Geometry: final body of the model. Coordinates: model frame, mm. Face numbers are marked on the shaded views. A direction names the side the tool comes from. Round coordinates to 2 decimals unless told otherwise and drop trailing zeros. Order: outer loops, then holes, each group sorted by start corner. A loop starts at its lowest first (then second) coordinate and runs counter-clockwise, first axis right, second up. Notation, with made-up numbers: (-5, 87) - (17, 87) arc R21 ccw to (17, 122) - close; hole circle Ø7 at (66, -33). An arc over 180 degrees is marked (long way). Put each result on its own line as item: value. Start each with the question number.
(1) Material intervals for L1, parallel to X at y = 3.35, z = 38.5; L2, parallel to Y at x = -114, z = 46.5; L3, parallel to X at y = 4, z = 41.25, sorted ascending. Write a range as [from, to].
(2) Section B-B (z = 43). Output: boundary loops of the cut face in (x, y).
(3) Pull-direction query (X, two-part tool) for the marked faces 3, 4 and 5; classes: released by +X, released by -X, zero draft, split by the parting line, or undercut.
(4) Section A-A (y = 3.95). Count the separate pieces of the cut face and the enclosed holes in it, and give its area (3 significant figures).
(5) Access query for the marked faces 1 and 2. Directions: +Z, -Z, +X, -X, +Y, -Y. A direction counts if a zero-diameter tool reaches every point of the face in a straight line with its end or side. Return the directions, or none.
(6) Pin query (flat end, axial travel): P1, Ø10, axis at x = -105, z = 35.5, coming from the +Y side. Return the tip coordinate at first contact, or that it passes through.
(7) Section C-C (x = -100). Output: boundary loops of the cut face in (y, z), and give its area (3 significant figures).
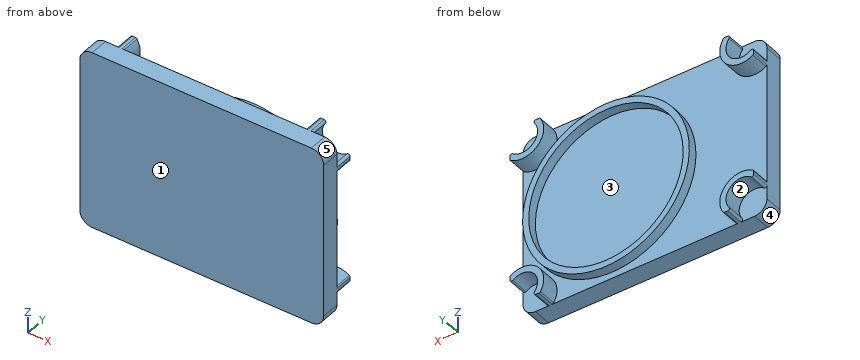
from build123d import *

# Parameters (mm, degrees)
SKETCH1_W           = 39.5
SKETCH1_H           = 29
BOSS_EXTRUDE1_DEPTH = 3
SKETCH2_R           = 13.5
SKETCH2_R_2         = 12.5
BOSS_EXTRUDE3_DEPTH = 1.5
BOSS_EXTRUDE4_DEPTH = 3
FILLET1_R           = 2
FILLET2_R           = 0.3


with BuildPart() as part:
    # Sketch1 → Boss-Extrude1 (new body)
    with BuildSketch(Plane(origin=(0, 0, 0), x_dir=(1, 0, 0), z_dir=(0, 1, 0))):
        with Locations((-109.95705295, -40.158748639)):
            Rectangle(SKETCH1_W, SKETCH1_H)
    extrude(amount=BOSS_EXTRUDE1_DEPTH)

    # Sketch2 → Boss-Extrude3 (add)
    with BuildSketch(Plane(origin=(0, 3, 0), x_dir=(1, 0, 0), z_dir=(0, 1, 0))):
        with Locations(Location((-104.70705295, -40.158748639, 0), (0, 0, 270))):
            Circle(SKETCH2_R)
        with Locations(Location((-104.70705295, -40.158748639, 0), (0, 0, 270))):
            Circle(SKETCH2_R_2, mode=Mode.SUBTRACT)
    extrude(amount=BOSS_EXTRUDE3_DEPTH)

    # Sketch3 → Boss-Extrude4 (add)
    with BuildSketch(Plane(origin=(0, 3, 0), x_dir=(1, 0, 0), z_dir=(0, 1, 0))):
        with BuildLine():
            Line((-124.834771627, -25.658748639), (-126.20705295, -25.658748639))
            ThreePointArc((-126.20705295, -25.658748639), (-125.939285997, -29.426515592), (-129.70705295, -29.158748639))
            Line((-129.70705295, -29.158748639), (-129.70705295, -30.531029962))
            ThreePointArc((-129.70705295, -30.531029962), (-125.232179216, -30.133622373), (-124.834771627, -25.658748639))
        make_face()
        with BuildLine():
            Line((-93.70705295, -25.658748639), (-95.079334273, -25.658748639))
            ThreePointArc((-95.079334273, -25.658748639), (-94.681926684, -30.133622373), (-90.20705295, -30.531029962))
            Line((-90.20705295, -30.531029962), (-90.20705295, -29.158748639))
            ThreePointArc((-90.20705295, -29.158748639), (-93.974819903, -29.426515592), (-93.70705295, -25.658748639))
        make_face()
        with BuildLine():
            ThreePointArc((-124.834771627, -54.658748639), (-125.232179216, -50.183874905), (-129.70705295, -49.786467316))
            Line((-129.70705295, -49.786467316), (-129.70705295, -51.158748639))
            ThreePointArc((-129.70705295, -51.158748639), (-125.939285997, -50.890981686), (-126.20705295, -54.658748639))
            Line((-126.20705295, -54.658748639), (-124.834771627, -54.658748639))
        make_face()
        with BuildLine():
            Line((-90.20705295, -51.158748639), (-90.20705295, -49.786467316))
            ThreePointArc((-90.20705295, -49.786467316), (-94.681926684, -50.183874905), (-95.079334273, -54.658748639))
            Line((-95.079334273, -54.658748639), (-93.70705295, -54.658748639))
            ThreePointArc((-93.70705295, -54.658748639), (-93.974819903, -50.890981686), (-90.20705295, -51.158748639))
        make_face()
    extrude(amount=BOSS_EXTRUDE4_DEPTH)

    # Fillet1
    fillet1_edges = [part.edges().sort_by_distance(p)[0] for p in [
        (-129.70705295, 1.5, 25.658748639),
        (-90.20705295, 1.5, 25.658748639),
        (-90.20705295, 1.5, 54.658748639),
        (-129.70705295, 1.5, 54.658748639),
    ]]
    fillet(fillet1_edges, radius=FILLET1_R)

    # Fillet2
    fillet2_edges = [part.edges().sort_by_distance(p)[0] for p in [
        (-93.70705295, 4.5, 54.658748639),
        (-90.20705295, 4.5, 51.158748639),
        (-90.20705295, 4.5, 49.786467316),
        (-95.079334273, 4.5, 54.658748639),
        (-126.20705295, 4.5, 54.658748639),
        (-124.834771627, 4.5, 54.658748639),
        (-129.70705295, 4.5, 49.786467316),
        (-129.70705295, 4.5, 51.158748639),
        (-93.70705295, 4.5, 25.658748639),
        (-95.079334273, 4.5, 25.658748639),
        (-90.20705295, 4.5, 30.531029962),
        (-90.20705295, 4.5, 29.158748639),
        (-129.70705295, 4.5, 29.158748639),
        (-129.70705295, 4.5, 30.531029962),
        (-124.834771627, 4.5, 25.658748639),
        (-126.20705295, 4.5, 25.658748639),
    ]]
    fillet(fillet2_edges, radius=FILLET2_R)


solid = part.part
Checks:
1. L1: x = [-118.1, -117.1], [-92.32, -91.31]
1. L2: y = [0, 3]
1. L3: x = [-118.16, -117.16], [-92.25, -91.25]
2. outline: (-129.71, 0) - (-90.21, 0) - (-90.21, 3) - (-91.51, 3) - (-91.51, 4.5) - (-92.53, 4.5) - (-92.53, 3) - (-116.88, 3) - (-116.88, 4.5) - (-117.9, 4.5) - (-117.9, 3) - (-129.71, 3) - close
3. face 3: undercut
3. face 4: released by -X
3. face 5: released by +X
4. separate pieces: 5
4. enclosed holes: 1
4. area: 117 mm²
5. face 1: +Z, -Z, +X, -X, -Y
5. face 2: +Y
6. P1: stops at y = 3
7. outline: (0, 25.66) - (3, 25.66) - (3, 27.51) - (4.5, 27.51) - (4.5, 28.58) - (3, 28.58) - (3, 51.74) - (4.5, 51.74) - (4.5, 52.81) - (3, 52.81) - (3, 54.66) - (0, 54.66) - close
7. area: 90.2 mm²
